Could you check a few things on this model? Use its own coordinates, in mm. A direction names the side the tool comes from. Round coordinates to 2 decimals unless told otherwise and drop trailing zeros. Write each loop counter-clockwise with the first axis right and the second up, starting at its lowest first coordinate (ties: lowest second). Pieces come first, ordered by that corner, then holes. Notation, with made-up numbers: M 55,26 L 70,26 A3 cw 70,30 Z; hole C 56,20.5 d4. An arc over 180 degrees is marked long. One line per item, written item: value. Start each with the question number.
(1) I want a section at C-C on x = 92. Please give me the cut outline in (y, z), and give its area (3 significant figures).
(2) If I drill on L1, parallel to X at y = 1.45, z = -52.5; L2, parallel to Y at x = 67.5, z = 2.25; L3, parallel to Y at x = 29.5, z = -42.5, over which ranges is the centre line in solid material (lowest first)?
(3) Thinking about a two-plate mould opening in Z: for faces 1 (the face through (53.31, 3.94, -11.96)), 2 (the face through (67, 49, -2)), 3 (the face through (85, 2, -60)), which applies, released by +Z, released by -Z, zero draft, split by the parting line, or undercut?
(4) Which directions (+Z, -Z, +X, -X, +Y, -Y) give clear straight access to the entire face, cutting with the end or side of a thin tool? Please do faces 4 (the face through (50, 8, -22)), 5 (the face through (73, 44, -2)), 6 (the face through (22.5, 86, 3)), 7 (the face through (26.5, 193, -52)).
(5) I'm going to push flat-ended pins straight in: pin 1 Ø1.8 at (x, z) = (85.25, -52.5) entering from +Y; pin 2 Ø10 at (y, z) = (157.5, -24) entering from +X; pin 3 Ø3.5 at (x, y) = (67.5, 43.5) entering from -Z; pin 4 Ø4.5 at (y, z) = (2.5, -51.5) entering from -X. Where does each tip first touch, or does it pass through?
(6) I want a section at A-A on x = 51. Please give me the cut outline in (y, z).
(7) I want a section at B-B on z = -56. Please give me the cut outline in (x, y).
```python
from build123d import *

# Parameters (mm, degrees)
PAD_DEPTH       = 6
SKETCH001_W     = 11
SKETCH001_H     = 11
PAD001_DEPTH    = 5
SKETCH003_R     = 1.5
POCKET_DEPTH    = 11.001
SKETCH004_R     = 1.5
POCKET001_DEPTH = 6
POCKET002_DEPTH = 6
SKETCH006_W     = 102
SKETCH006_H     = 8
PAD002_DEPTH    = 45
SKETCH007_W     = 35
SKETCH007_H     = 17.5
POCKET003_DEPTH = 4
SKETCH008_R     = 1.5
SKETCH008_W     = 8
SKETCH008_H     = 14.5
POCKET004_DEPTH = 5
SKETCH009_W     = 20
SKETCH009_H     = 4
PAD003_DEPTH    = 15
SKETCH010_R     = 1.5
POCKET005_DEPTH = 4
PAD004_DEPTH    = 45
SKETCH012_W     = 6
SKETCH012_H     = 6
PAD005_DEPTH    = 22
SKETCH013_W     = 20
SKETCH013_H     = 5
PAD006_DEPTH    = 15
SKETCH014_R     = 1.5
POCKET006_DEPTH = 195.001
SKETCH015_W     = 12
SKETCH015_H     = 35
PAD007_DEPTH    = 6
SKETCH016_R     = 1.5
POCKET007_DEPTH = 12.001
SKETCH018_R     = 2.5
POCKET008_DEPTH = 8
FILLET_R        = 2
FILLET001_R     = 2
FILLET002_R     = 2
FILLET003_R     = 2
FILLET004_R     = 2
FILLET005_R     = 2
FILLET006_R     = 2
FILLET007_R     = 1
FILLET008_R     = 2
FILLET009_R     = 2
FILLET010_R     = 2
FILLET011_R     = 1.5
FILLET012_R     = 2
FILLET013_R     = 2
POCKET009_DEPTH = 6


with BuildPart() as part:
    # Sketch → Pad (new body)
    with BuildSketch(Plane.XY):
        Polygon((0, 0), (102, 0), (102, 195), (69, 195), (69, 161), (33, 161), (33, 195), (0, 195), align=None)
    extrude(amount=PAD_DEPTH)

    # Sketch001 (on Face9 of Pad) → Pad001 (join)
    with BuildSketch(Plane(origin=(0, 0, 0), x_dir=(1, 0, 0), z_dir=(0, 0, -1))):
        with Locations((40.5, -43.5)):
            Rectangle(SKETCH001_W, SKETCH001_H)
        with Locations((67.5, -43.5)):
            Rectangle(SKETCH001_W, SKETCH001_H)
    extrude(amount=PAD001_DEPTH)

    # Sketch003 (on Face19 of Pad001) → Pocket (cut, through all)
    with BuildSketch(Plane(origin=(0, 0, -5), x_dir=(1, 0, 0), z_dir=(0, 0, -1))):
        with Locations((40.5, -43.5)):
            Circle(SKETCH003_R)
        with Locations((67.5, -43.5)):
            Circle(SKETCH003_R)
    extrude(amount=-POCKET_DEPTH, mode=Mode.SUBTRACT)

    # Sketch004 (on Face5 of Pocket) → Pocket001 (cut)
    with BuildSketch(Plane.XY.offset(6)):
        with Locations((21, 89.5)):
            Circle(SKETCH004_R)
        with Locations((81, 89.5)):
            Circle(SKETCH004_R)
        with Locations((81, 66.5)):
            Circle(SKETCH004_R)
        with Locations((21, 66.5)):
            Circle(SKETCH004_R)
    extrude(amount=-POCKET001_DEPTH, mode=Mode.SUBTRACT)

    # Sketch005 (on Face5 of Pocket001) → Pocket002 (cut)
    with BuildSketch(Plane.XY.offset(6)):
        Polygon((102, 185), (80, 185), (80, 163), (102, 163), (102, 168), (102, 180), align=None)
    extrude(amount=-POCKET002_DEPTH, mode=Mode.SUBTRACT)

    # Sketch006 (on Face4 of Pocket002) → Pad002 (join)
    with BuildSketch(Plane(origin=(0, 0, 0), x_dir=(1, 0, 0), z_dir=(0, 0, -1))):
        with Locations((51, -4)):
            Rectangle(SKETCH006_W, SKETCH006_H)
    extrude(amount=PAD002_DEPTH)

    # Sketch007 (on Face4 of Pad002) → Pocket003 (cut)
    with BuildSketch(Plane.XZ):
        with Locations((51, -36.25)):
            Rectangle(SKETCH007_W, SKETCH007_H)
    extrude(amount=-POCKET003_DEPTH, mode=Mode.SUBTRACT)

    # Sketch008 (on Face37 of Pocket003) → Pocket004 (cut)
    with BuildSketch(Plane.XZ.offset(-4)):
        with Locations((35.5, -29.5)):
            Circle(SKETCH008_R)
        with Locations((66.5, -29.5)):
            Circle(SKETCH008_R)
        with Locations((42.5, -37.75)):
            Rectangle(SKETCH008_W, SKETCH008_H)
    extrude(amount=-POCKET004_DEPTH, mode=Mode.SUBTRACT)

    # Sketch009 (on Face11 of Pocket004) → Pad003 (join)
    with BuildSketch(Plane(origin=(0, 0, -45), x_dir=(1, 0, 0), z_dir=(0, 0, -1))):
        with Locations((16.75, -2)):
            Rectangle(SKETCH009_W, SKETCH009_H)
        with Locations((85.25, -2)):
            Rectangle(SKETCH009_W, SKETCH009_H)
    extrude(amount=PAD003_DEPTH)

    # Sketch010 (on Face12 of Pad003) → Pocket005 (cut)
    with BuildSketch(Plane.XZ):
        with Locations((16.75, -52.5)):
            Circle(SKETCH010_R)
        with Locations((85.25, -52.5)):
            Circle(SKETCH010_R)
    extrude(amount=-POCKET005_DEPTH, mode=Mode.SUBTRACT)

    # Sketch011 (on Face7 of Pocket005) → Pad004 (join)
    with BuildSketch(Plane(origin=(0, 0, 0), x_dir=(1, 0, 0), z_dir=(0, 0, -1))):
        Polygon((96, -162), (102, -162), (102, -195), (69, -195), (69, -185), (96, -185), align=None)
        Polygon((0, -162), (6, -162), (6, -185), (33, -185), (33, -195), (0, -195), align=None)
    extrude(amount=PAD004_DEPTH)

    # Sketch012 (on Face25 of Pad004) → Pad005 (join)
    with BuildSketch(Plane.XZ.offset(-185)):
        with Locations((99, 3)):
            Rectangle(SKETCH012_W, SKETCH012_H)
    extrude(amount=PAD005_DEPTH)

    # Sketch013 (on Face37 of Pad005) → Pad006 (join)
    with BuildSketch(Plane(origin=(0, 0, -45), x_dir=(1, 0, 0), z_dir=(0, 0, -1))):
        with Locations((16.5, -192.5)):
            Rectangle(SKETCH013_W, SKETCH013_H)
        with Locations((85.5, -192.5)):
            Rectangle(SKETCH013_W, SKETCH013_H)
    extrude(amount=PAD006_DEPTH)

    # Sketch014 (on Face79 of Pad006) → Pocket006 (cut, through all)
    with BuildSketch(Plane(origin=(0, 195, 0), x_dir=(-1, 0, 0), z_dir=(0, 1, 0))):
        with Locations((-85.5, -52.5)):
            Circle(SKETCH014_R)
        with Locations((-16.5, -52.5)):
            Circle(SKETCH014_R)
    extrude(amount=-POCKET006_DEPTH, mode=Mode.SUBTRACT)

    # Sketch015 (on Face39 of Pocket006) → Pad007 (join)
    with BuildSketch(Plane(origin=(96, 0, 0), x_dir=(0, -1, 0), z_dir=(-1, 0, 0))):
        with Locations((-174, -11.5)):
            Rectangle(SKETCH015_W, SKETCH015_H)
    extrude(amount=PAD007_DEPTH)

    # Sketch016 (on Face92 of Pad007) → Pocket007 (cut, through all)
    with BuildSketch(Plane(origin=(90, 0, 0), x_dir=(0, -1, 0), z_dir=(-1, 0, 0))):
        with Locations((-174, -25)):
            Circle(SKETCH016_R)
    extrude(amount=-POCKET007_DEPTH, mode=Mode.SUBTRACT)

    # Sketch018 → Pocket008 (cut)
    with BuildSketch(Plane.XZ):
        with Locations((51, -11)):
            Circle(SKETCH018_R)
    extrude(amount=-POCKET008_DEPTH, mode=Mode.SUBTRACT)

    # Fillet
    fillet_edges = [part.edges().sort_by_distance(p)[0] for p in [
        (51, 0, 6),
    ]]
    fillet(fillet_edges, radius=FILLET_R)

    # Fillet001
    fillet001_edges = [part.edges().sort_by_distance(p)[0] for p in [
        (0, 98.5, 6),
        (102, 82.5, 6),
    ]]
    fillet(fillet001_edges, radius=FILLET001_R)

    # Fillet002
    fillet002_edges = [part.edges().sort_by_distance(p)[0] for p in [
        (102, 8, -22.5),
    ]]
    fillet(fillet002_edges, radius=FILLET002_R)

    # Fillet003
    fillet003_edges = [part.edges().sort_by_distance(p)[0] for p in [
        (0, 8, -22.5),
    ]]
    fillet(fillet003_edges, radius=FILLET003_R)

    # Fillet004
    fillet004_edges = [part.edges().sort_by_distance(p)[0] for p in [
        (33.5, 0, -36.25),
        (68.5, 0, -36.25),
    ]]
    fillet(fillet004_edges, radius=FILLET004_R)

    # Fillet005
    fillet005_edges = [part.edges().sort_by_distance(p)[0] for p in [
        (51, 0, -27.5),
    ]]
    fillet(fillet005_edges, radius=FILLET005_R)

    # Fillet006
    fillet006_edges = [part.edges().sort_by_distance(p)[0] for p in [
        (102, 162, -22.5),
    ]]
    fillet(fillet006_edges, radius=FILLET006_R)

    # Fillet007
    fillet007_edges = [part.edges().sort_by_distance(p)[0] for p in [
        (96, 162, -22.5),
    ]]
    fillet(fillet007_edges, radius=FILLET007_R)

    # Fillet008
    fillet008_edges = [part.edges().sort_by_distance(p)[0] for p in [
        (102, 195, -22.5),
        (69, 195, -22.5),
    ]]
    fillet(fillet008_edges, radius=FILLET008_R)

    # Fillet009
    fillet009_edges = [part.edges().sort_by_distance(p)[0] for p in [
        (51, 161, 6),
    ]]
    fillet(fillet009_edges, radius=FILLET009_R)

    # Fillet010
    fillet010_edges = [part.edges().sort_by_distance(p)[0] for p in [
        (33, 178, 6),
    ]]
    fillet(fillet010_edges, radius=FILLET010_R)

    # Fillet011
    fillet011_edges = [part.edges().sort_by_distance(p)[0] for p in [
        (69, 177, 6),
    ]]
    fillet(fillet011_edges, radius=FILLET011_R)

    # Fillet012
    fillet012_edges = [part.edges().sort_by_distance(p)[0] for p in [
        (33, 195, -22.5),
        (0, 195, -22.5),
    ]]
    fillet(fillet012_edges, radius=FILLET012_R)

    # Fillet013
    fillet013_edges = [part.edges().sort_by_distance(p)[0] for p in [
        (0, 162, -22.5),
        (6, 162, -22.5),
    ]]
    fillet(fillet013_edges, radius=FILLET013_R)

    # Sketch019 (on Face52 of Fillet013) → Pocket009 (cut)
    with BuildSketch(Plane.XY.offset(6)):
        with BuildLine():
            ThreePointArc((22.5, 106.5), (21, 108), (19.5, 106.5))
            Line((19.5, 106.5), (19.5, 66.5))
            ThreePointArc((19.5, 66.5), (21, 65), (22.5, 66.5))
            Line((22.5, 66.5), (22.5, 106.5))
        make_face()
        with BuildLine():
            ThreePointArc((82.5, 106.5), (81, 108), (79.5, 106.5))
            Line((79.5, 106.5), (79.5, 66.5))
            ThreePointArc((79.5, 66.5), (81, 65), (82.5, 66.5))
            Line((82.5, 66.5), (82.5, 106.5))
        make_face()
    extrude(amount=-POCKET009_DEPTH, mode=Mode.SUBTRACT)


solid = part.part
```
Found:
1. outline: M 0,-60 L 4,-60 L 4,-45 L 8,-45 L 8,0 L 163,0 L 163,6 L 2,6 A2 ccw 0,4 Z; M 168,-29 L 180,-29 L 180,6 L 168,6 Z; M 185,-45 L 190,-45 L 190,-60 L 195,-60 L 195,4 A2 ccw 193,6 L 185,6 Z; hole C 174,-25 d3
1. area: 2,390 mm²
2. L1: x = 6.75 to 15, 18.25 to 26.75, 75.25 to 83.75, 87 to 95.25
2. L2: y = 0 to 42, 45 to 161
2. L3: y = 0 to 8, 185 to 195
3. face 1: undercut
3. face 2: zero draft
3. face 3: released by -Z
4. face 4: -Z, +X, -X
4. face 5: -Z, +X
4. face 6: +Z, -Z
4. face 7: -Z, +Y
5. pin 1: passes through
5. pin 2: stops at x = 101.32
5. pin 3: stops at z = -5
5. pin 4: stops at x = 6.75
6. outline: M 0,-25.5 A2 ccw 2,-27.5 L 4,-27.5 L 4,-45 L 8,-45 L 8,-13.5 L 0,-13.5 Z; M 0,-8.5 L 8,-8.5 L 8,0 L 161,0 L 161,4 A2 ccw 159,6 L 2,6 A2 ccw 0,4 Z
7. outline: M 6.5,190 L 26.5,190 L 26.5,195 L 6.5,195 Z; M 6.75,0 L 26.75,0 L 26.75,4 L 6.75,4 Z; M 75.25,0 L 95.25,0 L 95.25,4 L 75.25,4 Z; M 75.5,190 L 95.5,190 L 95.5,195 L 75.5,195 Z
